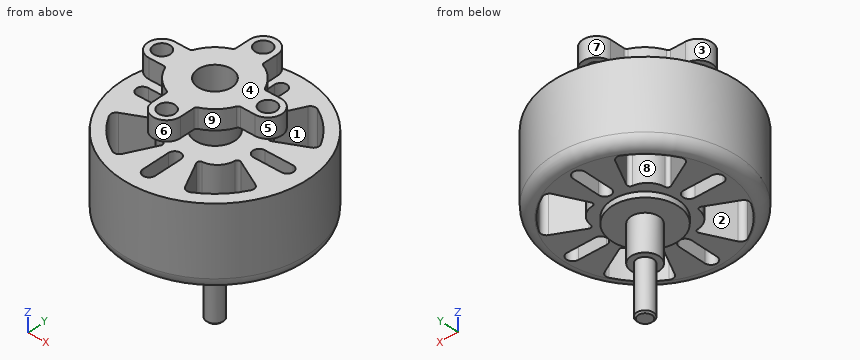
from build123d import *

# Parameters (mm, degrees)
IZIM1_R                     = 1.5
Y_KSEKLIK_EKSTR_ZYON1_DEPTH = 3.5
IZIM2_R                     = 4.444696269
Y_KSEKLIK_EKSTR_ZYON2_DEPTH = 5
Y_KSEKLIK_EKSTR_ZYON2_TAPER = 10
IZIM3_R                     = 16.6
Y_KSEKLIK_EKSTR_ZYON3_DEPTH = 14.3
IZIM4_R                     = 5.930506141
Y_KSEKLIK_EKSTR_ZYON4_DEPTH = 1
RADYUS1_R                   = 2
IZIM5_R                     = 2.5
Y_KSEKLIK_EKSTR_ZYON5_DEPTH = 15.5
IZIM7_R                     = 3.036237063
KES_EKSTR_ZYON1_DEPTH       = 15.5
KES_EKSTR_ZYON2_DEPTH       = 15.5
KES_EKSTR_ZYON3_DEPTH       = 14.3


# Read off the part's stored shape, not the designer's step: M3x0.5 Makine Dişleri Saplama1
with BuildPart() as part:
    # Çizim1 → Yükseklik-Ekstrüzyon1 (new body)
    with BuildSketch(Plane.XY):
        with BuildLine():
            Line((-6.873863542, 2.5), (-9.5, 2.5))
            ThreePointArc((-9.5, 2.5), (-12, 0), (-9.5, -2.5))
            Line((-9.5, -2.5), (-6.873863542, -2.5))
            ThreePointArc((-6.873863542, -2.5), (-6.600002264, -2.581669987), (-6.415605973, -2.8))
            ThreePointArc((-6.415605973, -2.8), (-4.949747468, -4.949747468), (-2.8, -6.415605973))
            ThreePointArc((-2.8, -6.415605973), (-2.581669987, -6.600002264), (-2.5, -6.873863542))
            Line((-2.5, -6.873863542), (-2.5, -9.5))
            ThreePointArc((-2.5, -9.5), (0, -12), (2.5, -9.5))
            Line((2.5, -9.5), (2.5, -6.873863542))
            ThreePointArc((2.5, -6.873863542), (2.581669987, -6.600002264), (2.8, -6.415605973))
            ThreePointArc((2.8, -6.415605973), (4.949747468, -4.949747468), (6.415605973, -2.8))
            ThreePointArc((6.415605973, -2.8), (6.600002264, -2.581669987), (6.873863542, -2.5))
            Line((6.873863542, -2.5), (9.5, -2.5))
            ThreePointArc((9.5, -2.5), (12, 0), (9.5, 2.5))
            Line((9.5, 2.5), (6.873863542, 2.5))
            ThreePointArc((6.873863542, 2.5), (6.600002264, 2.581669987), (6.415605973, 2.8))
            ThreePointArc((6.415605973, 2.8), (4.949747468, 4.949747468), (2.8, 6.415605973))
            ThreePointArc((2.8, 6.415605973), (2.581669987, 6.600002264), (2.5, 6.873863542))
            Line((2.5, 6.873863542), (2.5, 9.5))
            ThreePointArc((2.5, 9.5), (0, 12), (-2.5, 9.5))
            Line((-2.5, 9.5), (-2.5, 6.873863542))
            ThreePointArc((-2.5, 6.873863542), (-2.581669987, 6.600002264), (-2.8, 6.415605973))
            ThreePointArc((-2.8, 6.415605973), (-4.949747468, 4.949747468), (-6.415605973, 2.8))
            ThreePointArc((-6.415605973, 2.8), (-6.600002264, 2.581669987), (-6.873863542, 2.5))
        make_face()
        with Locations((0, -9.5)):
            Circle(IZIM1_R, mode=Mode.SUBTRACT)
        with Locations((9.5, 0)):
            Circle(IZIM1_R, mode=Mode.SUBTRACT)
        with Locations((-9.5, 0)):
            Circle(IZIM1_R, mode=Mode.SUBTRACT)
        with Locations((0, 9.5)):
            Circle(IZIM1_R, mode=Mode.SUBTRACT)
    extrude(amount=Y_KSEKLIK_EKSTR_ZYON1_DEPTH)

    # Çizim2 → Yükseklik-Ekstrüzyon2 (add)
    with BuildSketch(Plane(origin=(0, 0, 0), x_dir=(-1, 0, 0), z_dir=(0, 0, -1))):
        Circle(IZIM2_R)
    extrude(amount=Y_KSEKLIK_EKSTR_ZYON2_DEPTH, taper=Y_KSEKLIK_EKSTR_ZYON2_TAPER)

    # Çizim3 → Yükseklik-Ekstrüzyon3 (add)
    with BuildSketch(Plane(origin=(0, 0, -5), x_dir=(-1, 0, 0), z_dir=(0, 0, -1))):
        Circle(IZIM3_R)
    extrude(amount=Y_KSEKLIK_EKSTR_ZYON3_DEPTH)

    # Çizim4 → Yükseklik-Ekstrüzyon4 (add)
    with BuildSketch(Plane(origin=(0, 0, -19.3), x_dir=(-1, 0, 0), z_dir=(0, 0, -1))):
        Circle(IZIM4_R)
    extrude(amount=Y_KSEKLIK_EKSTR_ZYON4_DEPTH)

    # Radyus1
    radyus1_edges = [part.edges().sort_by_distance(p)[0] for p in [
        (16.6, 0, -19.3),
    ]]
    fillet(radyus1_edges, radius=RADYUS1_R)

    # Çizim5 → Yükseklik-Ekstrüzyon5 (add)
    with BuildSketch(Plane(origin=(0, 0, -20.3), x_dir=(-1, 0, 0), z_dir=(0, 0, -1))):
        Circle(IZIM5_R)
    extrude(amount=Y_KSEKLIK_EKSTR_ZYON5_DEPTH)

    # M3x0.5 Makine Dişleri Saplama1 outline → M3x0.5 Makine Dişleri Saplama1 (revolve, cut)
    with BuildSketch(Plane.XZ):
        Polygon((1.2195, -35.8), (2.5, -35.8), (2.5, -26.8), (1.5, -26.8), (1.5, -35.5195), align=None)
    revolve(axis=Axis((0, 0, 0), (0, 0, 1)), mode=Mode.SUBTRACT)

    # Çizim7 → Kes-Ekstrüzyon1 (cut)
    with BuildSketch(Plane.XY.offset(3.5)):
        Circle(IZIM7_R)
    extrude(amount=-KES_EKSTR_ZYON1_DEPTH, mode=Mode.SUBTRACT)

    # Çizim8 → Kes-Ekstrüzyon2 (cut)
    with BuildSketch(Plane.XY.offset(-5)):
        with BuildLine():
            Line((-7.354310006, 2.968244823), (-12.242132216, 5.473202633))
            ThreePointArc((-12.242132216, 5.473202633), (-12.741065417, 6.0665874), (-12.665995596, 6.838211883))
            ThreePointArc((-12.665995596, 6.838211883), (-10.277751926, 10.077519613), (-7.086052208, 12.529024315))
            ThreePointArc((-7.086052208, 12.529024315), (-6.305492258, 12.616142663), (-5.702755207, 12.112583838))
            Line((-5.702755207, 12.112583838), (-3.180498361, 7.162376053))
            ThreePointArc((-3.180498361, 7.162376053), (-3.188489381, 6.693341471), (-3.581591444, 6.437356972))
            ThreePointArc((-3.581591444, 6.437356972), (-5.663906626, 5.460279376), (-6.627977149, 3.371910354))
            ThreePointArc((-6.627977149, 3.371910354), (-6.883379112, 2.976172324), (-7.354310006, 2.968244823))
        make_face()
        with BuildLine():
            Line((2.968244823, 7.354310006), (5.473202633, 12.242132216))
            ThreePointArc((5.473202633, 12.242132216), (6.0665874, 12.741065417), (6.838211883, 12.665995596))
            ThreePointArc((6.838211883, 12.665995596), (10.077519613, 10.277751926), (12.529024315, 7.086052208))
            ThreePointArc((12.529024315, 7.086052208), (12.616142663, 6.305492258), (12.112583838, 5.702755207))
            Line((12.112583838, 5.702755207), (7.162376053, 3.180498361))
            ThreePointArc((7.162376053, 3.180498361), (6.693341471, 3.188489381), (6.437356972, 3.581591444))
            ThreePointArc((6.437356972, 3.581591444), (5.460279376, 5.663906626), (3.371910354, 6.627977149))
            ThreePointArc((3.371910354, 6.627977149), (2.976172324, 6.883379112), (2.968244823, 7.354310006))
        make_face()
        with BuildLine():
            Line((7.354310006, -2.968244823), (12.242132216, -5.473202633))
            ThreePointArc((12.242132216, -5.473202633), (12.741065417, -6.0665874), (12.665995596, -6.838211883))
            ThreePointArc((12.665995596, -6.838211883), (10.277751926, -10.077519613), (7.086052208, -12.529024315))
            ThreePointArc((7.086052208, -12.529024315), (6.305492258, -12.616142663), (5.702755207, -12.112583838))
            Line((5.702755207, -12.112583838), (3.180498361, -7.162376053))
            ThreePointArc((3.180498361, -7.162376053), (3.188489381, -6.693341471), (3.581591444, -6.437356972))
            ThreePointArc((3.581591444, -6.437356972), (5.663906626, -5.460279376), (6.627977149, -3.371910354))
            ThreePointArc((6.627977149, -3.371910354), (6.883379112, -2.976172324), (7.354310006, -2.968244823))
        make_face()
        with BuildLine():
            Line((-2.968244823, -7.354310006), (-5.473202633, -12.242132216))
            ThreePointArc((-5.473202633, -12.242132216), (-6.0665874, -12.741065417), (-6.838211883, -12.665995596))
            ThreePointArc((-6.838211883, -12.665995596), (-10.077519613, -10.277751926), (-12.529024315, -7.086052208))
            ThreePointArc((-12.529024315, -7.086052208), (-12.616142663, -6.305492258), (-12.112583838, -5.702755207))
            Line((-12.112583838, -5.702755207), (-7.162376053, -3.180498361))
            ThreePointArc((-7.162376053, -3.180498361), (-6.693341471, -3.188489381), (-6.437356972, -3.581591444))
            ThreePointArc((-6.437356972, -3.581591444), (-5.460279376, -5.663906626), (-3.371910354, -6.627977149))
            ThreePointArc((-3.371910354, -6.627977149), (-2.976172324, -6.883379112), (-2.968244823, -7.354310006))
        make_face()
    extrude(amount=-KES_EKSTR_ZYON2_DEPTH, mode=Mode.SUBTRACT)

    # Çizim9 → Kes-Ekstrüzyon3 (cut)
    with BuildSketch(Plane(origin=(0, 0, -19.3), x_dir=(-1, 0, 0), z_dir=(0, 0, -1))):
        with BuildLine():
            Line((-1.104517159, 7.922084558), (-1.104517159, 12.946929574))
            ThreePointArc((-1.104517159, 12.946929574), (0, 14.051446732), (1.104517159, 12.946929574))
            Line((1.104517159, 12.946929574), (1.104517159, 7.922084558))
            ThreePointArc((1.104517159, 7.922084558), (0, 6.8175674), (-1.104517159, 7.922084558))
        make_face()
        with BuildLine():
            Line((7.922084558, -1.104517159), (12.946929574, -1.104517159))
            ThreePointArc((12.946929574, -1.104517159), (14.051446732, 0), (12.946929574, 1.104517159))
            Line((12.946929574, 1.104517159), (7.922084558, 1.104517159))
            ThreePointArc((7.922084558, 1.104517159), (6.8175674, 0), (7.922084558, -1.104517159))
        make_face()
        with BuildLine():
            Line((-1.104517159, -7.922084558), (-1.104517159, -12.946929574))
            ThreePointArc((-1.104517159, -12.946929574), (0, -14.051446732), (1.104517159, -12.946929574))
            Line((1.104517159, -12.946929574), (1.104517159, -7.922084558))
            ThreePointArc((1.104517159, -7.922084558), (0, -6.8175674), (-1.104517159, -7.922084558))
        make_face()
        with BuildLine():
            Line((-7.922084558, 1.104517159), (-12.946929574, 1.104517159))
            ThreePointArc((-12.946929574, 1.104517159), (-14.051446732, 0), (-12.946929574, -1.104517159))
            Line((-12.946929574, -1.104517159), (-7.922084558, -1.104517159))
            ThreePointArc((-7.922084558, -1.104517159), (-6.8175674, 0), (-7.922084558, 1.104517159))
        make_face()
    extrude(amount=-KES_EKSTR_ZYON3_DEPTH, mode=Mode.SUBTRACT)


solid = part.part
The model under review builds one solid part; all positions refer to its coordinate system, in mm. Face numbers are marked on the shaded views. A direction names the side the tool comes from. Round coordinates to 2 decimals unless told otherwise and drop trailing zeros. Write each loop counter-clockwise with the first axis right and the second up, starting at its lowest first coordinate (ties: lowest second). Pieces come first, ordered by that corner, then holes. Notation, with made-up numbers: M -19,-34.75 L 22,-34.75 A22 ccw 22,-26.75 Z; hole C 70,-30.5 d6. An arc over 180 degrees is marked long. Answer as CSV lines item,"result". Start each with the question number.
Q1. Tool access review of the marked faces 5, 6, 7, 8 and 9: name each direction out of +Z, -Z, +X, -X, +Y, -Y from which nothing blocks a thin tool from reaching the whole face with its end or side.
Q2. Wall thickness on line 1 along Y through (x, z) = (0, 2); line 2 along Y through (x, z) = (-8.5, -16); line 3 along Z through (x, y) = (2.5, 4): over which ranges is each line inside the solid? List them lowest first.
Q3. The part is to be moulded in two halves that separate along Y. For the marked faces 1, 2, 3 and 4, say which applies: +Y half, -Y half, draft (parallel to the pull), parting line (faces both ways), or undercut.
Q4. Clearance check with flat-ended pins moving along their axes: P1, Ø10, axis at x = 5.5, z = -21.5, coming from the +Y side; P2, Ø3, axis at x = 1, y = 1, coming from the +Z side; P3, Ø1, axis at x = 11, y = 11.5, coming from the -Z side; P4, Ø12, axis at y = 12.5, z = -30.5, coming from the +X side. State where each tip first meets the part, or that it passes through.
Q5. Consider section A-A, the plane z = -16.5. State how many separate pieces and enclosed holes the cut face has, then the cut area to 3 significant figures.
Q6. Consider section D-D, the plane z = -4.5. Give the boundary of the cut face in (x, y), then the cut area to 3 significant figures.
Result set:
1,face 5,"+Z, +X"
1,face 6,"+Z, -Y"
1,face 7,"+Z, +Y"
1,face 8,"+Z, -Z"
1,face 9,"+Z, +X, -Y"
2,line 1,"y = -12 to -11, -8 to -3.04, 3.04 to 8, 11 to 12"
2,line 2,"y = -14.26 to -11.62, -3.86 to -1.1, 1.1 to 3.56, 11.62 to 14.26"
2,line 3,"z = -20.3 to -5, 0 to 3.5"
3,face 1,"undercut"
3,face 2,"undercut"
3,face 3,"parting line"
3,face 4,"draft"
4,P1,"stops at y = 16.41"
4,P2,"stops at z = -12"
4,P3,"stops at z = -19.13"
4,P4,"passes through"
5,separate pieces,"1"
5,enclosed holes,"8"
5,area,"591 mm²"
6,outline,"C 0,0 d7.3; hole C 0,0 d6.07"
6,area,"12.9 mm²"
